```python
from build123d import *

# Parameters (mm, degrees)
CROQUIS1_R              = 11
CROQUIS1_R_2            = 2
CROQUIS1_R_3            = 1.937672591
CROQUIS1_W              = 30
CROQUIS1_H              = 3
SALIENTE_EXTRUIR1_DEPTH = 3
CROQUIS2_R              = 13
CROQUIS2_R_2            = 11
SALIENTE_EXTRUIR2_DEPTH = 4
CROQUIS3_R              = 13
CROQUIS3_R_2            = 9
SALIENTE_EXTRUIR3_DEPTH = 2
CHAFL_N1_SIZE           = 2
CHAFL_N2_SIZE           = 10
CROQUIS4_W              = 10
CROQUIS4_H              = 20
CROQUIS4_R              = 2.5
SALIENTE_EXTRUIR4_DEPTH = 1.5


with BuildPart() as part:
    # Croquis1 → Saliente-Extruir1 (new body)
    with BuildSketch(Plane(origin=(0, 0, 0), x_dir=(1, 0, 0), z_dir=(0, 1, 0))):
        Polygon((-67.5, -20), (67.5, -20), (67.5, 20), (-67.5, 20), (-67.5, 10), (-57.5, 10), (-57.5, -10), (-67.5, -10), align=None)
        with Locations(Location((46.713951104, 0, 0), (0, 0, 270))):
            Circle(CROQUIS1_R, mode=Mode.SUBTRACT)
        with Locations(Location((-52.5, 0, 0), (0, 0, 270))):
            Circle(CROQUIS1_R_2, mode=Mode.SUBTRACT)
        with Locations(Location((27.185770037, 0, 0), (0, 0, 270))):
            Circle(CROQUIS1_R_3, mode=Mode.SUBTRACT)
        with Locations(Location((12.185770037, 0, 0), (0, 0, 270))):
            Circle(CROQUIS1_R_2, mode=Mode.SUBTRACT)
        with Locations((-27.5, 11)):
            Rectangle(CROQUIS1_W, CROQUIS1_H, mode=Mode.SUBTRACT)
        with Locations((-27.5, -11)):
            Rectangle(CROQUIS1_W, CROQUIS1_H, mode=Mode.SUBTRACT)
    extrude(amount=SALIENTE_EXTRUIR1_DEPTH)

    # Croquis2 → Saliente-Extruir2 (add)
    with BuildSketch(Plane(origin=(0, 3, 0), x_dir=(1, 0, 0), z_dir=(0, 1, 0))):
        with Locations(Location((46.713951104, 0, 0), (0, 0, 90))):
            Circle(CROQUIS2_R)
        with Locations(Location((46.713951104, 0, 0), (0, 0, 270))):
            Circle(CROQUIS2_R_2, mode=Mode.SUBTRACT)
    extrude(amount=SALIENTE_EXTRUIR2_DEPTH)

    # Croquis3 → Saliente-Extruir3 (add)
    with BuildSketch(Plane(origin=(0, 7, 0), x_dir=(1, 0, 0), z_dir=(0, 1, 0))):
        with Locations(Location((46.713951104, 0, 0), (0, 0, 90))):
            Circle(CROQUIS3_R)
        with Locations(Location((46.713951104, 0, 0), (0, 0, 270))):
            Circle(CROQUIS3_R_2, mode=Mode.SUBTRACT)
    extrude(amount=SALIENTE_EXTRUIR3_DEPTH)

    # Chaflán1
    chafl_n1_edges = [part.edges().sort_by_distance(p)[0] for p in [
        (46.713951104, 9, 13),
    ]]
    chamfer(chafl_n1_edges, length=CHAFL_N1_SIZE)

    # Chaflán2
    chafl_n2_edges = [part.edges().sort_by_distance(p)[0] for p in [
        (67.5, 1.5, 20),
        (67.5, 1.5, -20),
    ]]
    chamfer(chafl_n2_edges, length=CHAFL_N2_SIZE)

    # Croquis4 → Saliente-Extruir4 (add)
    with BuildSketch(Plane(origin=(0, 3, 0), x_dir=(1, 0, 0), z_dir=(0, 1, 0))):
        with Locations((-62.5, 0)):
            Rectangle(CROQUIS4_W, CROQUIS4_H)
        with Locations(Location((-62.5, 0, 0), (0, 0, 270))):
            Circle(CROQUIS4_R, mode=Mode.SUBTRACT)
    extrude(amount=-SALIENTE_EXTRUIR4_DEPTH)


solid = part.part
```
Check sheet for the modelled part. Datum: model origin and axes. Units: mm. A direction names the side the tool comes from. Coordinates: 2 decimals unless noted, no trailing zeros. Order: outer loops, then holes, each group sorted by start corner. A loop starts at its lowest first (then second) coordinate and runs counter-clockwise, first axis right, second up. Notation, with made-up numbers: M 45,85 L 86,85 A20 ccw 86,116 Z; hole C 81,-32.75 d5. An arc over 180 degrees is marked long. Write each question's results on one line, items separated by ' | '. Start each with the question number.
1. Cross-section at C-C on x = 31.5. Record the cut outline in (y, z).
2. Access from +Z, -Z, +X, -X, +Y, -Y to the whole of each face (thin tool, end or side, straight path). Record for faces 1 (the face through (-6, 1, 20)), 2 (the face through (-63.7, 1.5, -2.4)), 3 (the face through (55, 7, 4)), 4 (the face through (-42.5, 1, -11)).
3. Go/stop test with flat-tipped pins: P1, Ø10, axis at x = 31, z = 2, coming from the -Y side; P2, Ø20, axis at x = -18.5, z = -6.5, coming from the +Y side; P3, Ø5, axis at x = -62, z = 2, coming from the -Y side; P4, Ø2.5, axis at y = 1, z = 11.5, coming from the +X side. Record where each tip stops, or that it passes through.
4. Material ranges on probe 1 along Z at (x, y) = (-30.5, 1.75); probe 2 along X at (y, z) = (2.1, 0); probe 3 along Y at (x, z) = (-8.5, 4), recorded low to high.
5. Cross-section at B-B on z = 0. State how many separate pieces and enclosed holes the cut face has, and give its area (3 significant figures).
6. Mould release check, pull along X, two halves, no side actions. Record for faces 5 (the face through (-1, 0, 0)), 6 (the face through (-42.5, 1, 11)), 7 (the face through (62.4, 1.5, -15.1)), 8 (the face through (-64.72, 2.26, 1.15)): +X half, -X half, draft (parallel to the pull), parting line (faces both ways), or undercut.
7. Cross-section at D-D on y = 4.5. Record the cut outline in (x, z), and give its area (3 significant figures).
8. Cross-section at A-A on x = -62.5. Record the cut outline in (y, z), and give its area (3 significant figures).
Checks:
1) outline: M 0,-20 L 3,-20 L 3,20 L 0,20 Z
2) face 1: +Z, +X, -X, +Y, -Y | face 2: -X, -Y | face 3: -Y | face 4: +Y, -Y
3) P1: stops at y = 0 | P2: stops at y = 3 | P3: stops at y = 1.5 | P4: stops at x = 67.25
4) probe 1: z = -20 to -12.5, -9.5 to 9.5, 12.5 to 20 | probe 2: x = -67.5 to -65, -60 to -54.5, -50.5 to 10.19, 14.19 to 25.25, 29.12 to 35.71, 57.71 to 67.5 | probe 3: y = 0 to 3
5) separate pieces: 6 | enclosed holes: 0 | area: 309 mm²
6) face 5: draft | face 6: undercut | face 7: +X half | face 8: undercut
7) outline: C 46.71,0 d26; hole C 46.71,0 d22 | area: 151 mm²
8) outline: M 0,-20 L 3,-20 L 3,-2.5 L 1.5,-2.5 L 1.5,-10 L 0,-10 Z; M 0,10 L 1.5,10 L 1.5,2.5 L 3,2.5 L 3,20 L 0,20 Z | area: 82.5 mm²
